Source: CAD feature listing. Evaluate the final solid. Frame: model axes, mm. Face numbers are marked on the shaded views. Round coordinates to 2 decimals unless told otherwise and drop trailing zeros. Loops run counter-clockwise (first coordinate to the right, second up) from the corner with the lowest first, then second, coordinate; pieces in that order, holes last.
(1) First-contact query: pin 1 Ø3.5 at (x, z) = (29.5, 5) entering from +Y; pin 2 Ø13 at (x, y) = (44.5, 31) entering from +Z; pin 3 Ø0.9 at (y, z) = (31.5, 4.5) entering from +X; pin 4 Ø1 at (y, z) = (41, 2) entering from -X. Flat tips, straight axial feed; report the tip coordinate or a pass-through.
(2) Mould query, pull axis Y, two halves, no side actions, for the marked faces 1 and 2. Classes: pulls with the +Y half, pulls with the -Y half, needs draft (parallel to the pull), parting line crosses it, or undercut.
(3) Material intervals for probe 1 along X at (y, z) = (31, 5.25); probe 2 along Y at (x, z) = (51, 5.05); probe 3 along Z at (x, y) = (57, 14.5), sorted ascending.
(4) Section B-B, the plane y = 50. Return the cut outline in (x, z), plus the area to 3 significant figures.
(5) Section A-A, the plane x = 21. Return the cut outline in (y, z).
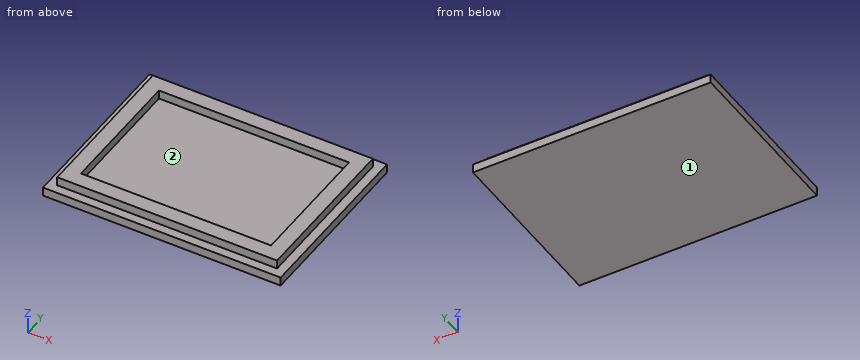
```python
from build123d import *

# Parameters (mm, degrees)
F0_W     = 64
F0_H     = 44
F1_DEPTH = 3
F0_W_2   = 80
F0_H_2   = 60
F0_W_3   = 74
F0_H_3   = 54
F2_DEPTH = 6


with BuildPart() as f1:
    # F0 (on Top) → F1 (new body)
    with BuildSketch(Plane.XY):
        with Locations((40, 30)):
            Rectangle(F0_W, F0_H)
    extrude(amount=F1_DEPTH)



with BuildPart() as f1b:
    # F0 (on Top) → F1, piece 2 (new body)
    with BuildSketch(Plane.XY):
        with Locations((40, 30)):
            Rectangle(F0_W_2, F0_H_2)
        with Locations((40, 30)):
            Rectangle(F0_W_3, F0_H_3, mode=Mode.SUBTRACT)
    extrude(amount=F1_DEPTH)


with BuildPart() as f1_1:
    add(f1.part)

    add(f1b.part)  # F2 merges F1b
    # F0 (on Top) → F2 (join)
    with BuildSketch(Plane.XY):
        with Locations((40, 30)):
            Rectangle(F0_W_3, F0_H_3)
        with Locations((40, 30)):
            Rectangle(F0_W, F0_H, mode=Mode.SUBTRACT)
    extrude(amount=F2_DEPTH)


solid = f1_1.part
```
Output values:
1. pin 1: stops at y = 57
1. pin 2: stops at z = 3
1. pin 3: stops at x = 77
1. pin 4: stops at x = 0
2. face 1: needs draft
2. face 2: undercut
3. probe 1: x = 3 to 8, 72 to 77
3. probe 2: y = 3 to 8, 52 to 57
3. probe 3: z = 0 to 3
4. outline: (0, 0) - (80, 0) - (80, 3) - (77, 3) - (77, 6) - (72, 6) - (72, 3) - (8, 3) - (8, 6) - (3, 6) - (3, 3) - (0, 3) - close
4. area: 270 mm2
5. outline: (0, 0) - (60, 0) - (60, 3) - (57, 3) - (57, 6) - (52, 6) - (52, 3) - (8, 3) - (8, 6) - (3, 6) - (3, 3) - (0, 3) - close
